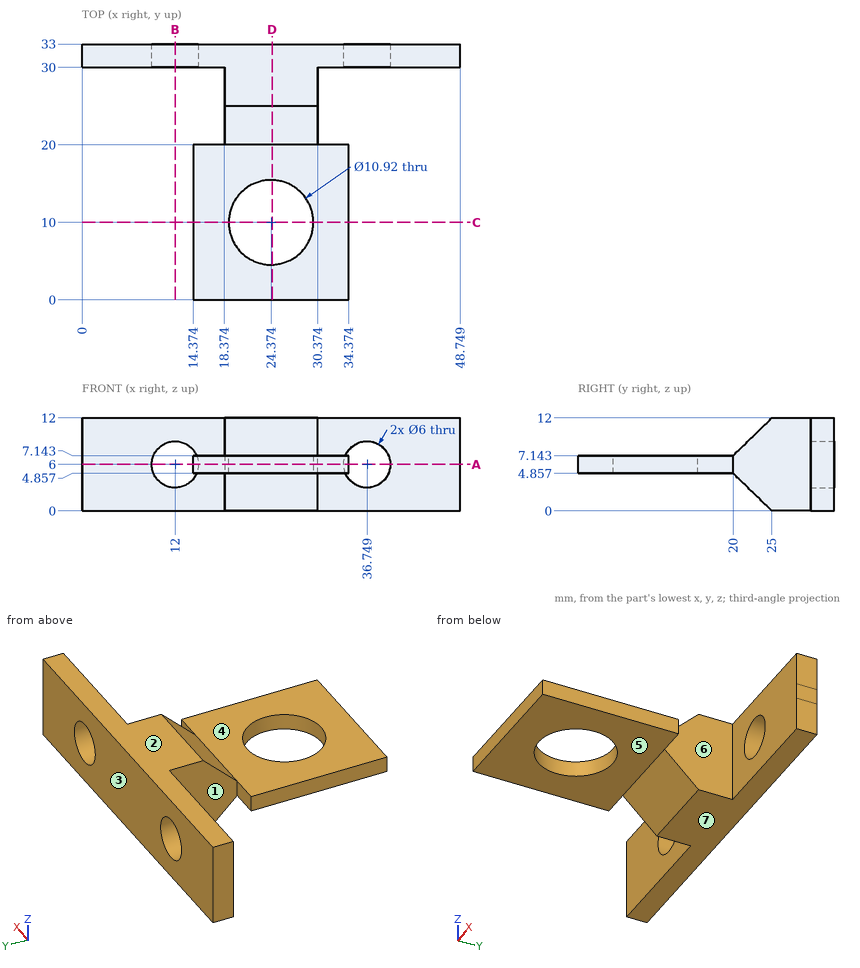
Geometry: see drawing. Coordinates: mm, zero at the bounding-box minimum. A direction names the side the tool comes from. Round coordinates to 2 decimals unless told otherwise and drop trailing zeros. Order: outer loops, then holes, each group sorted by start corner. A loop starts at its lowest first (then second) coordinate and runs counter-clockwise, first axis right, second up. Notation, with made-up numbers: (63.5, 89) -> (114.5, 89) arc R33 cw to (114.5, 122) -> close; hole circle Ø8 at (-17, 52.25). An arc over 180 degrees is marked (long way). Write each question's results on one line, items separated by ' | '.
Q1. Section query A-A (z = 6). Output: boundary loops of the cut face in (x, y) (1 decimal).
Response values:
outline: (0, 30) -> (9, 30) -> (9, 33) -> (0, 33) -> close; (14.4, 0) -> (34.4, 0) -> (34.4, 20) -> (30.4, 20) -> (30.4, 30) -> (33.7, 30) -> (33.7, 33) -> (15, 33) -> (15, 30) -> (18.4, 30) -> (18.4, 20) -> (14.4, 20) -> close; (39.7, 30) -> (48.7, 30) -> (48.7, 33) -> (39.7, 33) -> close; hole circle Ø10.9 at (24.4, 10)
Q2. Access query for the marked faces 4, 5, 6 and 7. Directions: +Z, -Z, +X, -X, +Y, -Y. A direction counts if a zero-diameter tool reaches every point of the face in a straight line with its end or side. Return the directions, or none.
Response values:
face 4: +Z, +X, -X, -Y | face 5: -Z, +X, -X, -Y | face 6: +Z, -Z, +X | face 7: -Z, +X, -X, +Y, -Y
Q3. Pin query (flat end, axial travel): pin 1 Ø5.5 at (x, z) = (12, 6) entering from +Y; pin 2 Ø3.5 at (x, z) = (36, 3.5) entering from -Y; pin 3 Ø1 at (x, y) = (31.5, 18.5) entering from -Z; pin 4 Ø5.5 at (x, z) = (36.75, 6) entering from -Y. Return the tip coordinate at first contact, or that it passes through.
Response values:
pin 1: y = 20 | pin 2: y = 30 | pin 3: z = 4.86 | pin 4: y = 0
Q4. Section query C-C (y = 10). Output: boundary loops of the cut face in (x, z) (1 decimal).
Response values:
outline: (14.4, 4.9) -> (18.9, 4.9) -> (18.9, 7.1) -> (14.4, 7.1) -> close; (29.8, 4.9) -> (34.4, 4.9) -> (34.4, 7.1) -> (29.8, 7.1) -> close
Q5. Pull-direction query (Y, two-part tool) for the marked faces 1, 2 and 3; classes: released by +Y, released by -Y, zero draft, split by the parting line, or undercut.
Response values:
face 1: undercut | face 2: zero draft | face 3: released by +Y
Q6. Ray query, line 1 along X through (y, z) = (32, 6); line 2 along Z through (x, y) = (12, 31); line 3 along Y through (x, z) = (8, 11.25). Return the intervals inside material, ascending.
Response values:
line 1: 0 to 9, 15 to 33.75, 39.75 to 48.75 | line 2: 0 to 3, 9 to 12 | line 3: 30 to 33
Q7. Section query B-B (x = 12). Output: boundary loops of the cut face in (y, z), and give its area (3 significant figures).
Response values:
outline: (30, 0) -> (33, 0) -> (33, 3) -> (30, 3) -> close; (30, 9) -> (33, 9) -> (33, 12) -> (30, 12) -> close | area: 18.0 mm²
Q8. Section query D-D (x = 24.5). Output: boundary loops of the cut face in (y, z).
Response values:
outline: (0, 4.86) -> (4.54, 4.86) -> (4.54, 7.14) -> (0, 7.14) -> close; (15.46, 4.86) -> (20, 4.86) -> (25, 0) -> (33, 0) -> (33, 12) -> (25, 12) -> (20, 7.14) -> (15.46, 7.14) -> close
